from build123d import *

# Parameters (mm, degrees)
CROQUIS1_W              = 80
CROQUIS1_H              = 60
CROQUIS1_R              = 1.5
CROQUIS1_W_2            = 7
CROQUIS1_H_2            = 25
CROQUIS1_W_3            = 10
CROQUIS1_H_3            = 20
CROQUIS1_H_4            = 10
CROQUIS1_W_4            = 5
CROQUIS1_H_5            = 6.5
SALIENTE_EXTRUIR1_DEPTH = 15
CORTAR_EXTRUIR1_DEPTH   = 10
CROQUIS3_R              = 1.5
CORTAR_EXTRUIR2_DEPTH   = 25
CORTAR_EXTRUIR3_START   = -25
CROQUIS6_R              = 1.5
CORTAR_EXTRUIR3_DEPTH   = 25
CROQUIS8_W              = 15
CROQUIS8_H              = 17.838651154
CROQUIS8_R              = 1.5
SALIENTE_EXTRUIR2_DEPTH = 5
CORTAR_EXTRUIR4_START   = -55
CORTAR_EXTRUIR4_DEPTH   = 8
CROQUIS10_R             = 1.5
CROQUIS10_W             = 7
CROQUIS10_H             = 12
CORTAR_EXTRUIR5_DEPTH   = 16
CROQUIS12_W             = 110
CROQUIS12_H             = 15
SALIENTE_EXTRUIR3_DEPTH = 3
CORTAR_EXTRUIR6_DEPTH   = 10
SALIENTE_EXTRUIR4_DEPTH = 15
CROQUIS15_R             = 2.25
CORTAR_EXTRUIR7_DEPTH   = 10
CORTAR_EXTRUIR8_START   = -10
CROQUIS16_R             = 2.25
CORTAR_EXTRUIR8_DEPTH   = 10


with BuildPart() as part:
    # Croquis1 → Saliente-Extruir1 (new body)
    # profile 1 of 13: a face of its own
    with BuildSketch(Plane(origin=(0, 0, 0), x_dir=(1, 0, 0), z_dir=(0, 1, 0))):
        with Locations((0, -10)):
            Rectangle(CROQUIS1_W, CROQUIS1_H)
        with Locations(Location((18, -16.5, 0), (0, 0, 270))):
            Circle(CROQUIS1_R, mode=Mode.SUBTRACT)
        with Locations(Location((-11, -16.5, 0), (0, 0, 270))):
            Circle(CROQUIS1_R, mode=Mode.SUBTRACT)
        with Locations(Location((18, 16.5, 0), (0, 0, 270))):
            Circle(CROQUIS1_R, mode=Mode.SUBTRACT)
        with Locations(Location((-11, 16.5, 0), (0, 0, 270))):
            Circle(CROQUIS1_R, mode=Mode.SUBTRACT)
        with Locations((18, 0)):
            Rectangle(CROQUIS1_W_2, CROQUIS1_H_2, mode=Mode.SUBTRACT)
        Polygon((6.711696879, 3.875), (0, 7.75), (-6.711696879, 3.875), (-6.711696879, -3.875), (0, -7.75), (6.711696879, -3.875), align=None, mode=Mode.SUBTRACT)
        with Locations((-11, 0)):
            Rectangle(CROQUIS1_W_2, CROQUIS1_H_2, mode=Mode.SUBTRACT)
    # profile 2 of 13: a face of its own
    with BuildSketch(Plane(origin=(0, 0, 0), x_dir=(1, 0, 0), z_dir=(0, 1, 0))):
        with Locations((-45, -10)):
            Rectangle(CROQUIS1_W_3, CROQUIS1_H_3)
    # profile 3 of 13: a face of its own
    with BuildSketch(Plane(origin=(0, 0, 0), x_dir=(1, 0, 0), z_dir=(0, 1, 0))):
        with Locations((-45, -35)):
            Rectangle(CROQUIS1_W_3, CROQUIS1_H_4)
    # profile 4 of 13: a face of its own
    with BuildSketch(Plane(origin=(0, 0, 0), x_dir=(1, 0, 0), z_dir=(0, 1, 0))):
        with Locations((-52.5, -10)):
            Rectangle(CROQUIS1_W_4, CROQUIS1_H)
    # profile 5 of 13: a face of its own
    with BuildSketch(Plane(origin=(0, 0, 0), x_dir=(1, 0, 0), z_dir=(0, 1, 0))):
        with Locations((-45, 15)):
            Rectangle(CROQUIS1_W_3, CROQUIS1_H_4)
    # profile 6 of 13: a face of its own
    with BuildSketch(Plane(origin=(0, 0, 0), x_dir=(1, 0, 0), z_dir=(0, 1, 0))):
        with Locations((45, 15)):
            Rectangle(CROQUIS1_W_3, CROQUIS1_H_4)
    # profile 7 of 13: a face of its own
    with BuildSketch(Plane(origin=(0, 0, 0), x_dir=(1, 0, 0), z_dir=(0, 1, 0))):
        with Locations((52.5, -10)):
            Rectangle(CROQUIS1_W_4, CROQUIS1_H)
    # profile 8 of 13: a face of its own
    with BuildSketch(Plane(origin=(0, 0, 0), x_dir=(1, 0, 0), z_dir=(0, 1, 0))):
        with Locations((45, -10)):
            Rectangle(CROQUIS1_W_3, CROQUIS1_H_3)
    # profile 9 of 13: a face of its own
    with BuildSketch(Plane(origin=(0, 0, 0), x_dir=(1, 0, 0), z_dir=(0, 1, 0))):
        with Locations((45, -35)):
            Rectangle(CROQUIS1_W_3, CROQUIS1_H_4)
    # profile 10 of 13: a face of its own
    with BuildSketch(Plane(origin=(0, 0, 0), x_dir=(1, 0, 0), z_dir=(0, 1, 0))):
        with Locations((-11, 9.25)):
            Rectangle(CROQUIS1_W_2, CROQUIS1_H_5)
    # profile 11 of 13: a face of its own
    with BuildSketch(Plane(origin=(0, 0, 0), x_dir=(1, 0, 0), z_dir=(0, 1, 0))):
        with Locations((-11, -9.25)):
            Rectangle(CROQUIS1_W_2, CROQUIS1_H_5)
    # profile 12 of 13: a face of its own
    with BuildSketch(Plane(origin=(0, 0, 0), x_dir=(1, 0, 0), z_dir=(0, 1, 0))):
        with Locations((18, 9.25)):
            Rectangle(CROQUIS1_W_2, CROQUIS1_H_5)
    # profile 13 of 13: a face of its own
    with BuildSketch(Plane(origin=(0, 0, 0), x_dir=(1, 0, 0), z_dir=(0, 1, 0))):
        with Locations((18, -9.25)):
            Rectangle(CROQUIS1_W_2, CROQUIS1_H_5)
    extrude(amount=SALIENTE_EXTRUIR1_DEPTH)

    # Croquis2 → Cortar-Extruir1 (cut)
    with BuildSketch(Plane.XZ):
        Polygon((-7.391560818, 16.5), (-9.195780409, 19.625), (-12.804219591, 19.625), (-14.608439182, 16.5), (-12.804219591, 13.375), (-9.195780409, 13.375), align=None)
        Polygon((21.608439182, 16.5), (19.804219591, 19.625), (16.195780409, 19.625), (14.391560818, 16.5), (16.195780409, 13.375), (19.804219591, 13.375), align=None)
        Polygon((-7.391560818, -16.5), (-9.195780409, -13.375), (-12.804219591, -13.375), (-14.608439182, -16.5), (-12.804219591, -19.625), (-9.195780409, -19.625), align=None)
        Polygon((21.608439182, -16.5), (19.804219591, -13.375), (16.195780409, -13.375), (14.391560818, -16.5), (16.195780409, -19.625), (19.804219591, -19.625), align=None)
    extrude(amount=-CORTAR_EXTRUIR1_DEPTH, mode=Mode.SUBTRACT)

    # Croquis3 → Cortar-Extruir2 (cut)
    with BuildSketch(Plane(origin=(55, 0, 0), x_dir=(0, 0, -1), z_dir=(1, 0, 0))):
        with Locations((-25, 7.5)):
            Circle(CROQUIS3_R)
        with Locations((5, 7.5)):
            Circle(CROQUIS3_R)
    extrude(amount=-CORTAR_EXTRUIR2_DEPTH, mode=Mode.SUBTRACT)

    # Croquis6 → Cortar-Extruir3 (cut)
    with BuildSketch(Plane.ZY.offset(55).offset(CORTAR_EXTRUIR3_START)):
        with Locations(Location((-5, 7.5, 0), (0, 0, 180))):
            Circle(CROQUIS6_R)
        with Locations(Location((25, 7.5, 0), (0, 0, 180))):
            Circle(CROQUIS6_R)
    extrude(amount=CORTAR_EXTRUIR3_DEPTH, mode=Mode.SUBTRACT)

    # Croquis8 → Saliente-Extruir2 (add)
    with BuildSketch(Plane(origin=(0, 15, 0), x_dir=(1, 0, 0), z_dir=(0, 1, 0))):
        Rectangle(CROQUIS8_W, CROQUIS8_H)
        with Locations(Location((0, 0, 0), (0, 0, 270))):
            Circle(CROQUIS8_R, mode=Mode.SUBTRACT)
    extrude(amount=-SALIENTE_EXTRUIR2_DEPTH)

    # Croquis9 → Cortar-Extruir4 (cut, symmetric)
    with BuildSketch(Plane(origin=(55, 0, 0), x_dir=(0, 0, -1), z_dir=(1, 0, 0)).offset(CORTAR_EXTRUIR4_START)):
        Polygon((-40, 3), (-12.5, 15), (-40, 15), align=None)
    extrude(amount=CORTAR_EXTRUIR4_DEPTH, both=True, mode=Mode.SUBTRACT)

    # Croquis10 → Cortar-Extruir5 (cut)
    with BuildSketch(Plane(origin=(0, 15, 0), x_dir=(1, 0, 0), z_dir=(0, 1, 0))):
        with Locations(Location((25, -12, 0), (0, 0, 270))):
            Circle(CROQUIS10_R)
        with Locations(Location((25, -36, 0), (0, 0, 270))):
            Circle(CROQUIS10_R)
        with Locations((25, -24)):
            Rectangle(CROQUIS10_W, CROQUIS10_H)
    extrude(amount=-CORTAR_EXTRUIR5_DEPTH, mode=Mode.SUBTRACT)

    # Croquis12 → Saliente-Extruir3 (add)
    with BuildSketch(Plane(origin=(0, 0, -20), x_dir=(-1, 0, 0), z_dir=(0, 0, -1))):
        with Locations((0, 7.5)):
            Rectangle(CROQUIS12_W, CROQUIS12_H)
    extrude(amount=SALIENTE_EXTRUIR3_DEPTH)

    # Croquis13 → Cortar-Extruir6 (cut)
    with BuildSketch(Plane.XZ):
        Polygon((28.608439182, 12), (26.804219591, 15.125), (23.195780409, 15.125), (21.391560818, 12), (23.195780409, 8.875), (26.804219591, 8.875), align=None)
        Polygon((28.608439182, 36), (26.804219591, 39.125), (23.195780409, 39.125), (21.391560818, 36), (23.195780409, 32.875), (26.804219591, 32.875), align=None)
    extrude(amount=-CORTAR_EXTRUIR6_DEPTH, mode=Mode.SUBTRACT)

    # Croquis14 → Saliente-Extruir4 (add)
    with BuildSketch(Plane.XZ):
        with BuildLine():
            Line((30, 41), (30, 42))
            ThreePointArc((30, 42), (29.707106781, 42.707106781), (29, 43))
            Line((29, 43), (21, 43))
            ThreePointArc((21, 43), (20.292893219, 42.707106781), (20, 42))
            Line((20, 42), (20, 41))
            ThreePointArc((20, 41), (19.707106781, 40.292893219), (19, 40))
            Line((19, 40), (31, 40))
            ThreePointArc((31, 40), (30.292893219, 40.292893219), (30, 41))
        make_face()
    extrude(amount=-SALIENTE_EXTRUIR4_DEPTH)

    # Croquis15 → Cortar-Extruir7 (cut)
    with BuildSketch(Plane(origin=(55, 0, 0), x_dir=(0, 0, -1), z_dir=(1, 0, 0))):
        with Locations((-25, 7.5)):
            Circle(CROQUIS15_R)
        with Locations((5, 7.5)):
            Circle(CROQUIS15_R)
    extrude(amount=-CORTAR_EXTRUIR7_DEPTH, mode=Mode.SUBTRACT)

    # Croquis16 → Cortar-Extruir8 (cut)
    with BuildSketch(Plane.ZY.offset(55).offset(CORTAR_EXTRUIR8_START)):
        with Locations(Location((-5, 7.5, 0), (0, 0, 180))):
            Circle(CROQUIS16_R)
        with Locations(Location((25, 7.5, 0), (0, 0, 180))):
            Circle(CROQUIS16_R)
    extrude(amount=CORTAR_EXTRUIR8_DEPTH, mode=Mode.SUBTRACT)


solid = part.part
Design review of the part built by this model. Coordinates are the model's own, in mm. A direction names the side the tool comes from. Give positions to 0.01 mm unless a question says otherwise; leave off trailing zeros. Order: outer loops, then holes, each group sorted by start corner. A loop starts at its lowest first (then second) coordinate and runs counter-clockwise, first axis right, second up.
1. Add section C-C, the plane x = -11. State the section outline as (y, z) points (3 decimals), then the cut area to 3 significant figures.
Solution:
outline: (0, -23) - (15, -23) - (15, -18) - (10, -18) - (10, -19.625) - (0, -19.625) - close; (0, -13.375) - (10, -13.375) - (10, -15) - (15, -15) - (15, -6) - (0, -6) - close; (0, 6) - (15, 6) - (15, 15) - (10, 15) - (10, 13.375) - (0, 13.375) - close; (0, 19.625) - (10, 19.625) - (10, 18) - (15, 18) - (15, 40) - (0, 40) - close
area: 610 mm2
2. Mouldability with a two-part tool opening along Y and no side actions: class faces 1 (the flat face through (43, 7, 40)), 2 (the flat face through (20, 10, 17)), 3 (the cylindrical face through (-52.465, 6.824, 22.854)), 4 (the cylindrical face through (35.1, 6.6, 26.2)) as +Y half, -Y half, draft (parallel to the pull), parting line (faces both ways), or undercut.
Solution:
face 1: draft
face 2: -Y half
face 3: undercut
face 4: undercut
3. Add section B-B, the plane x = -45. State the section outline as (y, z) points, then the cut area to 3 significant figures.
Solution:
outline: (0, -23) - (15, -23) - (15, -10) - (0, -10) - close; (0, 0) - (15, 0) - (15, 20) - (0, 20) - close; (0, 30) - (15, 30) - (15, 40) - (0, 40) - close
area: 645 mm2
4. Tool access review of faces 5 (the flat face through (55, 7, 9)), 6 (the flat face through (45, 7, 30)), 7 (the cylindrical face through (52.535, 9.397, -6.21)), 8 (the flat face through (27.694, 4.93, 34.416)): name each direction out of +Z, -Z, +X, -X, +Y, -Y from which nothing blocks a thin tool from reaching the whole face with its end or side.
Solution:
face 5: +Z, -Z, +X, +Y, -Y
face 6: +Y, -Y
face 7: +X
face 8: -Y
5. Add section A-A, the plane x = 25. State the section outline as (y, z) points (3 decimals), then the cut area to 3 significant figures.
Solution:
outline: (0, -23) - (15, -23) - (15, 10.5) - (10, 10.5) - (10, 8.875) - (0, 8.875) - close; (0, 15.125) - (10, 15.125) - (10, 13.5) - (15, 13.5) - (15, 18) - (0, 18) - close; (0, 30) - (15, 30) - (15, 34.5) - (10, 34.5) - (10, 32.875) - (0, 32.875) - close; (0, 39.125) - (10, 39.125) - (10, 37.5) - (15, 37.5) - (15, 43) - (0, 43) - close
area: 655 mm2
6. Add section D-D, the plane z = 25. State how many separate pieces and enclosed holes the cut face has, then the cut area to 3 significant figures.
Solution:
separate pieces: 6
enclosed holes: 0
area: 1,050 mm2
7. To check wall thickness, follow L1, parallel to X at y = 13.75, z = 25.5; L2, parallel to X at y = 2, z = 20.5; L3, parallel to X at y = 13.75, z = 16.5. State the ranges of each line that lie inside material, in increasing order.
Solution:
L1: x = -55 to -50, -40 to -8, 8 to 21.5, 28.5 to 40, 50 to 55
L2: x = -55 to -50, -40 to 21.5, 28.5 to 40, 50 to 55
L3: x = -55 to -12.5, -9.5 to -8, 8 to 16.5, 19.5 to 55
8. For pin 1 Ø2 at (x, y) = (18, 6.5) entering from +Z; pin 2 Ø1 at (x, y) = (0.5, 6.5) entering from +Z (3 decimals); pin 3 Ø7.5 at (x, y) = (-4, 11) entering from +Z; pin 4 Ø2.5 at (x, z) = (-11, -16.5) entering from -Y, all flat-tipped, find the tip position at first contact; note any pin that passes through.
Solution:
pin 1: stops at z = 40
pin 2: stops at z = 33.125
pin 3: stops at z = 30.26
pin 4: passes through
